The figure shows three views and two pictorial views of one solid part (mm, origin at its lowest corner). Answer the questions. Coordinates: 2 decimals unless noted, no trailing zeros. Loops run counter-clockwise (first coordinate to the right, second up) from the corner with the lowest first, then second, coordinate; pieces in that order, holes last. Notation, with made-up numbers: M -8,58.25 L 25,58.25 A27 cw 25,76.25 Z; hole C -37.75,82 d6. An arc over 180 degrees is marked long. One line per item, written item: value. Start each with the question number.
1. Flat-ended cylindrical pins translate along their axes: pin 1 (3 mm diameter, centred on x = 1, z = 4.5, fed in from -Y); pin 2 (2.5 mm diameter, centred on x = 2.8, y = 2.8, fed in from -Z); pin 3 (2.5 mm diameter, centred on x = 2.5, y = 2.5, fed in from -Z). Find the tip coordinate at first contact, or state that the pin passes through.
2. The part is cut by section B-B (z = 4.5). Write down the section's boundary in (x, y), then the cut area to 3 significant figures.
3. The part is cut by section D-D (z = 12). Write down the section's boundary in (x, y).
4. Consider probe 1 along Y at (x, z) = (2.8, 38.4); probe 2 along X at (y, z) = (2.7, 11); probe 3 along Y at (x, z) = (3.65, 36.5). Determine where each line is inside the solid, lowest interval first.
5. The part is cut by section A-A (y = 2.8). Write down the section's boundary in (x, z).
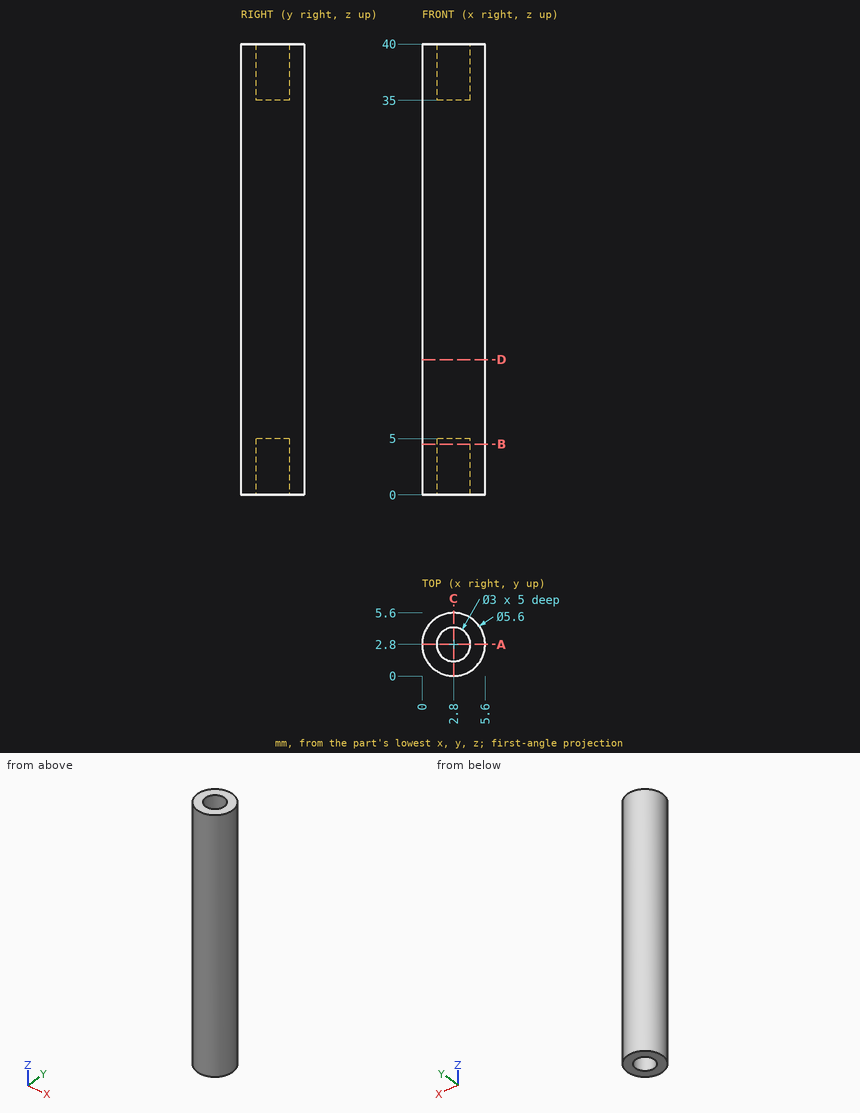
Answer block:
1. pin 1: stops at y = 0.02
1. pin 2: stops at z = 5
1. pin 3: stops at z = 0
2. outline: C 2.8,2.8 d5.6; hole C 2.8,2.8 d3
2. area: 17.6 mm2
3. outline: C 2.8,2.8 d5.6
4. probe 1: y = 0 to 1.3, 4.3 to 5.6
4. probe 2: x = 0 to 5.6
4. probe 3: y = 0.13 to 1.56, 4.04 to 5.47
5. outline: M 0,0 L 1.3,0 L 1.3,5 L 4.3,5 L 4.3,0 L 5.6,0 L 5.6,40 L 4.3,40 L 4.3,35 L 1.3,35 L 1.3,40 L 0,40 Z
